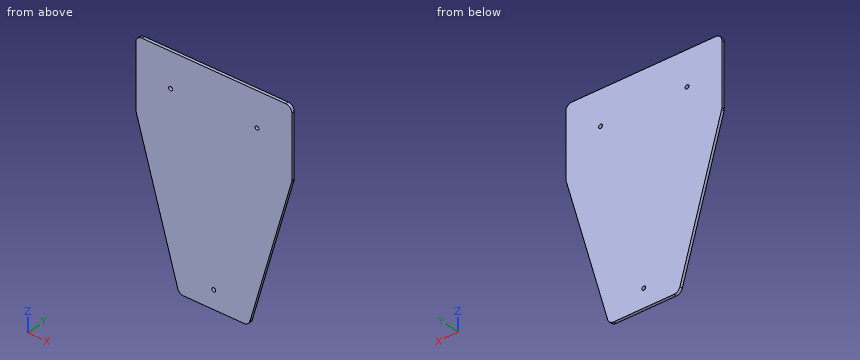
```python
from build123d import *

# Parameters (mm, degrees)
BOSS_EXTRUDE1_DEPTH = 2.36
FILLET1_R           = 5
SKETCH4_R           = 1.5625
CUT_EXTRUDE1_DEPTH  = 3.36


with BuildPart() as part:
    # Sketch3 → Boss-Extrude1 (new body)
    with BuildSketch(Plane(origin=(0, 0, 0), x_dir=(1, 0, 0), z_dir=(0, 1, 0))):
        Polygon((-63.18, -28.18), (63.18, -28.18), (63.18, 28.18), (28.18, 151.82), (-28.18, 151.82), (-63.18, 28.18), align=None)
    extrude(amount=BOSS_EXTRUDE1_DEPTH)

    # Fillet1
    fillet1_edges = [part.edges().sort_by_distance(p)[0] for p in [
        (63.18, 1.18, -28.18),
        (63.18, 1.18, 28.18),
        (-63.18, 1.18, 28.18),
        (-63.18, 1.18, -28.18),
        (-28.18, 1.18, -151.82),
        (28.18, 1.18, -151.82),
    ]]
    fillet(fillet1_edges, radius=FILLET1_R)

    # Sketch4 → Cut-Extrude1 (cut, through all)
    with BuildSketch(Plane(origin=(0, 2.36, 0), x_dir=(1, 0, 0), z_dir=(0, 1, 0))):
        with Locations((-35, 0)):
            Circle(SKETCH4_R)
        with Locations((35, 0)):
            Circle(SKETCH4_R)
        with Locations((0, 136.82)):
            Circle(SKETCH4_R)
    extrude(amount=-CUT_EXTRUDE1_DEPTH, mode=Mode.SUBTRACT)


solid = part.part
```
Here's how the part is built. I have some questions about the finished solid (model axes, mm). Give positions to 0.01 mm unless a question says otherwise; leave off trailing zeros. Loops run counter-clockwise (first coordinate to the right, second up) from the corner with the lowest first, then second, coordinate; pieces in that order, holes last. Notation, with made-up numbers: M 82.25,-38.5 L 99.25,-38.5 A19 cw 99.25,-25.5 Z; hole C 46.25,-1.75 d5. An arc over 180 degrees is marked long. Return JSON: item names as keys, results as strings.
Item 1: Please list where these lines run through material, in increasing order: line 1 (X direction, y = 1.75, z = 0); line 2 (Z direction, x = 0, y = 1.8); line 3 (X direction, y = 1.15, z = -136.82).
A:
{"line 1": "x = -63.18 to -36.56, -33.44 to 33.44, 36.56 to 63.18", "line 2": "z = -151.82 to -138.38, -135.26 to 28.18", "line 3": "x = -32.43 to -1.56, 1.56 to 32.43"}
Item 2: Imagine slicing it at A-A on y = 0.9. List the corners of the cut face in (x, z) for me (1 decimal), then the cut area to 3 significant figures.
A:
{"outline": "M -63.2,-27.5 A5 ccw -63,-28.8 L -29.2,-148.2 A5 ccw -24.4,-151.8 L 24.4,-151.8 A5 ccw 29.2,-148.2 L 63,-28.8 A5 ccw 63.2,-27.5 L 63.2,23.2 A5 ccw 58.2,28.2 L -58.2,28.2 A5 ccw -63.2,23.2 Z; hole C -35,0 d3.1; hole C 0,-136.8 d3.1; hole C 35,0 d3.1", "area": "18,400 mm^2"}
Item 3: Imagine slicing it at C-C on x = -43.5. List the corners of the cut face in (y, z) for me, then the cut area to 3 significant figures.
A:
{"outline": "M 0,-97.7 L 2.36,-97.7 L 2.36,28.18 L 0,28.18 Z", "area": "297 mm^2"}
Item 4: Imagine slicing it at B-B on z = -54. List the corners of the cut face in (x, y) for me.
A:
{"outline": "M -55.87,0 L 55.87,0 L 55.87,2.36 L -55.87,2.36 Z"}
